```python
from build123d import *

# Parameters (mm, degrees)
SKETCH1_W           = 139.192
SKETCH1_H           = 177.292
BOSS_EXTRUDE1_DEPTH = 6.35
SKETCH2_W           = 6.55
SKETCH2_H           = 177.292
CUT_EXTRUDE1_DEPTH  = 3.375
SKETCH5_R           = 2.286
CUT_EXTRUDE3_DEPTH  = 12.7


with BuildPart() as part:
    # Sketch1 → Boss-Extrude1 (new body)
    with BuildSketch(Plane(origin=(0, 0, 0), x_dir=(1, 0, 0), z_dir=(0, 1, 0))):
        with Locations((69.596, 88.646)):
            Rectangle(SKETCH1_W, SKETCH1_H)
    extrude(amount=BOSS_EXTRUDE1_DEPTH)

    # Sketch2 → Cut-Extrude1 (cut)
    with BuildSketch(Plane(origin=(0, 6.35, 0), x_dir=(1, 0, 0), z_dir=(0, 1, 0))):
        with Locations((135.917, 88.646)):
            Rectangle(SKETCH2_W, SKETCH2_H)
        with Locations((3.275, 88.646)):
            Rectangle(SKETCH2_W, SKETCH2_H)
    extrude(amount=-CUT_EXTRUDE1_DEPTH, mode=Mode.SUBTRACT)

    # Sketch5 → Cut-Extrude3 (cut)
    with BuildSketch(Plane.XZ):
        with Locations((107.188, -10.414)):
            Circle(SKETCH5_R)
        with Locations((97.282, -10.414)):
            Circle(SKETCH5_R)
        with Locations((41.91, -10.414)):
            Circle(SKETCH5_R)
        with Locations((32.004, -10.414)):
            Circle(SKETCH5_R)
    extrude(amount=-CUT_EXTRUDE3_DEPTH, mode=Mode.SUBTRACT)


solid = part.part
```
Check sheet for the modelled part. Datum: model origin and axes. Units: mm. A direction names the side the tool comes from. Round coordinates to 2 decimals unless told otherwise and drop trailing zeros. Loops run counter-clockwise (first coordinate to the right, second up) from the corner with the lowest first, then second, coordinate; pieces in that order, holes last. Notation, with made-up numbers: (-20.5, 60.25) - (-4.5, 60.25) arc R33 ccw to (-4.5, 91.25) - close; hole circle Ø11 at (84.5, 83.25). An arc over 180 degrees is marked (long way). Answer as a JSON object with one key per item and string values. Group by question number.
Q1. Sectioned sample at A-A, the plane x = 41.91. Enter the section's corners in (y, z).
Q2. Sectioned sample at B-B, the plane z = -164.5. Enter the section's corners in (x, y) (3 decimals), plus the area to 3 significant figures.
Q3. Gauge pin test, flat ends, axial feed: P1, Ø4, axis at x = 97.282, z = -10.414, coming from the -Y side; P2, Ø1, axis at y = 5, z = -75, coming from the -X side; P3, Ø7, axis at x = 137, z = -124, coming from the +Y side (3 decimals); P4, Ø1, axis at y = 5.5, z = -130, coming from the +X side. Record the tip position at first contact, or that the pin passes through.
Q4. Mould release check, pull along Z, two halves, no side actions. Record for faces 1 (the face through (95.597, 3.131, -8.869)), 2 (the face through (3, 2.975, -90)), 3 (the face through (109.37, 3.13, -9.73)), 4 (the face through (69, 3, -177.292)): released by +Z, released by -Z, zero draft, split by the parting line, or undercut.
Q5. Set-up check for faces 5 (the face through (136, 2.975, -90)), 6 (the face through (69, 6.35, -90)): record each of +Z, -Z, +X, -X, +Y, -Y from which the full face is reachable in a straight line by a thin tool's end or side.
Q6. Scan lines: line 1 along X through (y, z) = (4.75, -40); line 2 along Z through (x, y) = (41.91, 3.25); line 3 along Z through (x, y) = (43, 1.75). Record each from-to range of solid material in increasing order. Write a range as [from, to].
Solution:
{
 "1": {"outline": "(0, -177.29) - (6.35, -177.29) - (6.35, -12.7) - (0, -12.7) - close; (0, -8.13) - (6.35, -8.13) - (6.35, 0) - (0, 0) - close"},
 "2": {"outline": "(0, 0) - (139.192, 0) - (139.192, 2.975) - (132.642, 2.975) - (132.642, 6.35) - (6.55, 6.35) - (6.55, 2.975) - (0, 2.975) - close", "area": "840 mm²"},
 "3": {"P1": "passes through", "P2": "stops at x = 6.55", "P3": "stops at y = 2.975", "P4": "stops at x = 132.64"},
 "4": {"face 1": "undercut", "face 2": "zero draft", "face 3": "undercut", "face 4": "released by -Z"},
 "5": {"face 5": "+Z, -Z, +X, +Y", "face 6": "+Z, -Z, +X, -X, +Y"},
 "6": {"line 1": "x = [6.55, 132.64]", "line 2": "z = [-177.29, -12.7], [-8.13, 0]", "line 3": "z = [-177.29, -12.42], [-8.4, 0]"}
}
